```python
from build123d import *

# Parameters (mm, degrees)
F0_R     = 22.5
F0_R_2   = 20
F1_DEPTH = 3
F2_R     = 20
F2_R_2   = 17.5
F3_DEPTH = 0.5


# Not quite as in the source:
# - a pattern or mirror of a feature is missing from the dataset's text; its kind, count and spacing are read off the source's solid


with BuildPart() as f1:
    # F0 (on Front) → F1 (new body, symmetric)
    with BuildSketch(Plane.XZ):
        Circle(F0_R)
        Circle(F0_R_2, mode=Mode.SUBTRACT)
    extrude(amount=F1_DEPTH, both=True)

    # F2 (on face) → F3 (join)
    with BuildSketch(Plane.XZ.offset(3)):
        Circle(F2_R)
        Circle(F2_R_2, mode=Mode.SUBTRACT)
    f3 = extrude(amount=-F3_DEPTH)

    # F3_copies: F3 across plane
    add(f3.mirror(Plane.ZX))


solid = f1.part
```
Read the model definition and answer for the solid it produces. Units are mm, in the model's axes. A direction names the side the tool comes from. Give positions to 0.01 mm unless a question says otherwise; leave off trailing zeros. Order: outer loops, then holes, each group sorted by start corner. A loop starts at its lowest first (then second) coordinate and runs counter-clockwise, first axis right, second up. Notation, with made-up numbers: (29.25, -12) -> (40.25, -12) arc R18 ccw to (40.25, 14) -> close; hole circle Ø2 at (-10, 5). An arc over 180 degrees is marked (long way). One line per item, written item: value. Start each with the question number.
(1) For a pull along Z with two mould halves and no side action, classify faces 1 (the flat face through (12, 3, -13)), 2 (the cylindrical face through (10.382, -0.042, -19.961)), 3 (the flat face through (0, 2.5, -18)) as released by +Z, released by -Z, zero draft, split by the parting line, or undercut.
(2) The part is cut by section C-C (y = 0.7). Determine the outline of the cut face in (x, z), and give its area (3 significant figures).
(3) Straight lines are drawn through the part: L1, parallel to Z at x = 0, y = -2.8; L2, parallel to Y at x = -5, z = -17; L3, parallel to Z at x = 0, y = 0.55. For each, find the intervals that lie inside material, in ascending order.
(4) The part is cut by section D-D (x = 19). Determine the outline of the cut face in (y, z) (3 decimals), and give its area (3 significant figures).
(5) A tool of negligible diameter and unlimited length cuts with its end or side. For faces 4 (the cylindrical face through (-13.887, 2.754, -10.648)), 5 (the flat face through (0, -2.5, -18)), from which of +Z, -Z, +X, -X, +Y, -Y can it reach the whole face along a straight path? Write none if from no direction.
(6) The part is cut by section A-A (z = 0). Determine the outline of the cut face in (x, y), and give its area (3 significant figures).
(7) Flat-ended cylindrical pins translate along their axes: P1, Ø3, axis at x = -3.5, y = -2.5, coming from the -Z side; P2, Ø3, axis at x = -0.5, y = 1.5, coming from the +Z side; P3, Ø3, axis at x = 3, y = -0.5, coming from the +Z side. Find the tip coordinate at first contact, or state that the pin passes through.
(8) The part is cut by section B-B (x = 0). Determine the outline of the cut face in (y, z).
Taken from the geometry:
1. face 1: zero draft
1. face 2: split by the parting line
1. face 3: undercut
2. outline: circle Ø45 at (0, 0); hole circle Ø40 at (0, 0)
2. area: 334 mm^2
3. L1: -22.5 to -17.5, 17.5 to 22.5
3. L2: -3 to -2.5, 2.5 to 3
3. L3: -22.5 to -20, 20 to 22.5
4. outline: (-3, -12.052) -> (3, -12.052) -> (3, 12.052) -> (-3, 12.052) -> close; hole (-2.5, -6.245) -> (2.5, -6.245) -> (2.5, 6.245) -> (-2.5, 6.245) -> close
4. area: 82.2 mm^2
5. face 4: +Y, -Y
5. face 5: none
6. outline: (-22.5, -3) -> (-17.5, -3) -> (-17.5, -2.5) -> (-20, -2.5) -> (-20, 2.5) -> (-17.5, 2.5) -> (-17.5, 3) -> (-22.5, 3) -> close; (17.5, -3) -> (22.5, -3) -> (22.5, 3) -> (17.5, 3) -> (17.5, 2.5) -> (20, 2.5) -> (20, -2.5) -> (17.5, -2.5) -> close
6. area: 35.0 mm^2
7. P1: z = -22.41
7. P2: z = 22.5
7. P3: z = 22.45
8. outline: (-3, -22.5) -> (3, -22.5) -> (3, -17.5) -> (2.5, -17.5) -> (2.5, -20) -> (-2.5, -20) -> (-2.5, -17.5) -> (-3, -17.5) -> close; (-3, 17.5) -> (-2.5, 17.5) -> (-2.5, 20) -> (2.5, 20) -> (2.5, 17.5) -> (3, 17.5) -> (3, 22.5) -> (-3, 22.5) -> close
